Autodesk Inventor part; units mm, degrees
ref_plane "YZ Plane" through (0, 0, 0) normal (1, 0, 0) x (0, 1, 0)
ref_plane "XZ Plane" through (0, 0, 0) normal (0, 1, 0) x (-1, 0, 0)
ref_plane "XY Plane" through (0, 0, 0) normal (0, 0, 1) x (1, 0, 0)
sketch "Sketch1" plane through (0, 0, 0) normal (0, 1, 0) x (-1, 0, 0)
  line L0 (0, 0) -> (12.7, 0)
  line L1 (12.7, 0) -> (12.7, -12.7)
  line L2 (12.7, -12.7) -> (0, -12.7)
  line L3 (0, -12.7) -> (0, 0)
  dimension "d0" = 12.7
  dimension "d1" = 12.7
extrude "Extrusion1" add sketch "Sketch1" along normal blind 3.175
sketch "Sketch2" plane through (0, 3.175, 0) normal (0, 1, 0) x (1, 0, 0)
  line L0 (-12.7, 12.7) -> (-12.7, 0)
  line L1 (0, 0) -> (-12.7, 0)
  line L2 (-12.7, 0) -> (-12.7, 3.175)
  line L3 (-12.7, 3.175) -> (0, 3.175)
  line L4 (0, 3.175) -> (0, 0)
  dimension "d4" = 3.175
extrude "Extrusion2" add sketch "Sketch2" along normal blind 25.4
sketch "Sketch3" plane through (-12.7, 0, 0) normal (0, 0, 1) x (1, 0, 0)
  circle A0 centre (6.35, 20.32) radius 3.175
  line L0 (12.7, 0) -> (0, 0)
  line L1 (0, 0) -> (0, 28.575)
  dimension "d7" = 6.35
  dimension "d8" = 20.32
  dimension "d9" = 6.35
extrude "Extrusion3" cut sketch "Sketch3" against normal blind 4.7625
properties part number "BackMount2CylinderAdapter"
Design review of the part built by this model. Coordinates are the model's own, in mm. A direction names the side the tool comes from. Round coordinates to 2 decimals unless told otherwise and drop trailing zeros. Write each loop counter-clockwise with the first axis right and the second up, starting at its lowest first coordinate (ties: lowest second). Pieces come first, ordered by that corner, then holes.
Item 1: Consider section C-C on z = -1.25. Give the boundary of the cut face in (x, y) (3 decimals).
Item 2: Consider section A-A on x = -6.35. Give the boundary of the cut face in (y, z) (3 decimals).
Item 3: For faces 5 (the flat face through (-6, 2, -12.7)), 6 (the flat face through (-6, 16, -3.175)), list the 3-axis set-ups (+Z, -Z, +X, -X, +Y, -Y) from which the entire face can be reached by the end or side of a thin tool; tool diameter is ignored.
Item 4: For pin 1 Ø5 at (x, y) = (-4, 8) entering from -Z (3 decimals), flat-tipped, find the tip position at first contact; note if it passes through.
Item 5: Consider section B-B on y = 20.32. Give the boundary of the cut face in (x, z) (3 decimals), and give its area (3 significant figures).
Item 6: Wall thickness on L1, parallel to Y at x = -6.35, z = -0.7 (3 decimals); L2, parallel to Z at x = -0.75, y = 12.25 (3 decimals); L3, parallel to Y at x = -8, z = -9.25 (3 decimals): over which ranges is each line inside the solid? List them lowest first.
Item 7: Draft analysis for pull direction X (two halves, no side actions). For faces 1 (the cylindrical face through (-3.32, 21.27, -1.57)), 2 (the flat face through (0, 11, -3)), 3 (the flat face through (-12.7, 11, -3)), 4 (the flat face through (-6, 3.175, -8)), state which applies: released by +X, released by -X, zero draft, split by the parting line, or undercut.
Item 8: Consider section D-D on x = -11. Give the boundary of the cut face in (y, z) (3 decimals).
Check values:
1. outline: (-12.7, 0) - (0, 0) - (0, 28.575) - (-12.7, 28.575) - close; hole circle Ø6.35 at (-6.35, 20.32)
2. outline: (0, -12.7) - (3.175, -12.7) - (3.175, -3.175) - (17.145, -3.175) - (17.145, 0) - (0, 0) - close; (23.495, -3.175) - (28.575, -3.175) - (28.575, 0) - (23.495, 0) - close
3. face 5: -Z, +X, -X, +Y, -Y
3. face 6: -Z, +X, -X, +Y
4. pin 1: stops at z = -3.175
5. outline: (-12.7, -3.175) - (-9.525, -3.175) - (-9.525, 0) - (-12.7, 0) - close; (-3.175, -3.175) - (0, -3.175) - (0, 0) - (-3.175, 0) - close
5. area: 20.2 mm2
6. L1: y = 0 to 17.145, 23.495 to 28.575
6. L2: z = -3.175 to 0
6. L3: y = 0 to 3.175
7. face 1: undercut
7. face 2: released by +X
7. face 3: released by -X
7. face 4: zero draft
8. outline: (0, -12.7) - (3.175, -12.7) - (3.175, -3.175) - (28.575, -3.175) - (28.575, 0) - (0, 0) - close
